from build123d import *

# Parameters (mm, degrees)
SKETCH1_W              = 250
SKETCH1_H              = 80
CARD_BASE_DEPTH        = 10
SKETCH3_W              = 5
SKETCH3_H              = 50
F_2BRIDGE_HOLDER_DEPTH = 10
SKETCH5_W              = 5
SKETCH5_H              = 50
F_3BRIDGE_HOLDER_DEPTH = 10
SKETCH6_W              = 5
SKETCH6_H              = 50
F_4BRIDGE_HOLDER_DEPTH = 10
SKETCH7_W              = 5
SKETCH7_H              = 50
F_5BRIDGE_HOLDER_DEPTH = 10
SKETCH8_W              = 5
SKETCH8_H              = 50
F_6BRIDGE_HOLDER_DEPTH = 10
SKETCH9_W              = 5
SKETCH9_H              = 50
F_7_BH_DEPTH           = 10
SKETCH10_W             = 5
SKETCH10_H             = 50
F_8BH_DEPTH            = 10
SKETCH11_W             = 5
SKETCH11_H             = 50
F_9BH_DEPTH            = 10
SKETCH12_W             = 5
SKETCH12_H             = 50
F_10BH_DEPTH           = 10
SKETCH13_W             = 5
SKETCH13_H             = 50
F_11BH_DEPTH           = 10


with BuildPart() as part:
    # Sketch1 → Card Base (new body)
    with BuildSketch(Plane(origin=(0, 0, 0), x_dir=(1, 0, 0), z_dir=(0, 1, 0))):
        with Locations((-0.650367763, 0.037958261)):
            Rectangle(SKETCH1_W, SKETCH1_H)
    extrude(amount=CARD_BASE_DEPTH)

    # Sketch3 → 2bridge holder (cut)
    with BuildSketch(Plane(origin=(0, 10, 0), x_dir=(1, 0, 0), z_dir=(0, 1, 0))):
        with Locations((-118.150367763, 0.037958261)):
            Rectangle(SKETCH3_W, SKETCH3_H)
    extrude(amount=-F_2BRIDGE_HOLDER_DEPTH, mode=Mode.SUBTRACT)

    # Sketch5 → 3bridge holder (cut)
    with BuildSketch(Plane(origin=(0, 10, 0), x_dir=(1, 0, 0), z_dir=(0, 1, 0))):
        with Locations((-93.150367763, 0.037958261)):
            Rectangle(SKETCH5_W, SKETCH5_H)
    extrude(amount=-F_3BRIDGE_HOLDER_DEPTH, mode=Mode.SUBTRACT)

    # Sketch6 → 4Bridge holder (cut)
    with BuildSketch(Plane(origin=(0, 10, 0), x_dir=(1, 0, 0), z_dir=(0, 1, 0))):
        with Locations((-68.150367763, 0.037958261)):
            Rectangle(SKETCH6_W, SKETCH6_H)
    extrude(amount=-F_4BRIDGE_HOLDER_DEPTH, mode=Mode.SUBTRACT)

    # Sketch7 → 5Bridge holder (cut)
    with BuildSketch(Plane(origin=(0, 10, 0), x_dir=(1, 0, 0), z_dir=(0, 1, 0))):
        with Locations((-43.150367763, 0.037958261)):
            Rectangle(SKETCH7_W, SKETCH7_H)
    extrude(amount=-F_5BRIDGE_HOLDER_DEPTH, mode=Mode.SUBTRACT)

    # Sketch8 → 6bridge holder (cut)
    with BuildSketch(Plane(origin=(0, 10, 0), x_dir=(1, 0, 0), z_dir=(0, 1, 0))):
        with Locations((-18.150367763, 0.037958261)):
            Rectangle(SKETCH8_W, SKETCH8_H)
    extrude(amount=-F_6BRIDGE_HOLDER_DEPTH, mode=Mode.SUBTRACT)

    # Sketch9 → 7 BH (cut)
    with BuildSketch(Plane(origin=(0, 10, 0), x_dir=(1, 0, 0), z_dir=(0, 1, 0))):
        with Locations((6.849632237, 0.037958261)):
            Rectangle(SKETCH9_W, SKETCH9_H)
    extrude(amount=-F_7_BH_DEPTH, mode=Mode.SUBTRACT)

    # Sketch10 → 8BH (cut)
    with BuildSketch(Plane(origin=(0, 10, 0), x_dir=(1, 0, 0), z_dir=(0, 1, 0))):
        with Locations((31.849632237, 0.037958261)):
            Rectangle(SKETCH10_W, SKETCH10_H)
    extrude(amount=-F_8BH_DEPTH, mode=Mode.SUBTRACT)

    # Sketch11 → 9BH (cut)
    with BuildSketch(Plane(origin=(0, 10, 0), x_dir=(1, 0, 0), z_dir=(0, 1, 0))):
        with Locations((56.849632237, 0.037958261)):
            Rectangle(SKETCH11_W, SKETCH11_H)
    extrude(amount=-F_9BH_DEPTH, mode=Mode.SUBTRACT)

    # Sketch12 → 10BH (cut)
    with BuildSketch(Plane(origin=(0, 10, 0), x_dir=(1, 0, 0), z_dir=(0, 1, 0))):
        with Locations((81.849632237, 0.037958261)):
            Rectangle(SKETCH12_W, SKETCH12_H)
    extrude(amount=-F_10BH_DEPTH, mode=Mode.SUBTRACT)

    # Sketch13 → 11BH (cut)
    with BuildSketch(Plane(origin=(0, 10, 0), x_dir=(1, 0, 0), z_dir=(0, 1, 0))):
        with Locations((106.849632237, 0.037958261)):
            Rectangle(SKETCH13_W, SKETCH13_H)
    extrude(amount=-F_11BH_DEPTH, mode=Mode.SUBTRACT)


solid = part.part
Check sheet for the modelled part. Datum: model origin and axes. Units: mm. Give positions to 0.01 mm unless a question says otherwise; leave off trailing zeros. Loops run counter-clockwise (first coordinate to the right, second up) from the corner with the lowest first, then second, coordinate; pieces in that order, holes last. Notation, with made-up numbers: M -33.5,49.5 L -20.5,49.5 A23 ccw -20.5,81.5 Z; hole C 19,54 d10. An arc over 180 degrees is marked long. Return JSON: item names as keys, results as strings. Group by question number.
1. Cross-section at A-A on x = -93. Record the boundary of the cut face in (y, z), plus the area to 3 significant figures.
2. Mould release check, pull along X, two halves, no side actions. Record for faces 1 (the flat face through (-2, 0, -1)), 2 (the flat face through (-95.65, 5, 0)): released by +X, released by -X, zero draft, split by the parting line, or undercut.
3. Cross-section at B-B on z = -16.5. State how many separate pieces and enclosed holes the cut face has, plus the area to 3 significant figures.
4. Thickness scan on L1, parallel to Z at x = -94.5, y = 2.5. Record the ranges inside material, lowest first.
Return value:
{
 "1": {"outline": "M 0,-40.04 L 10,-40.04 L 10,-25.04 L 0,-25.04 Z; M 0,24.96 L 10,24.96 L 10,39.96 L 0,39.96 Z", "area": "300 mm^2"},
 "2": {"face 1": "zero draft", "face 2": "undercut"},
 "3": {"separate pieces": "11", "enclosed holes": "0", "area": "2,000 mm^2"},
 "4": {"L1": "-40.04 to -25.04, 24.96 to 39.96"}
}
